Print and shaded views of the part. All mm, measured from the part's lowest x, y and z. Coordinates: 2 decimals unless noted, no trailing zeros. Loops run counter-clockwise (first coordinate to the right, second up) from the corner with the lowest first, then second, coordinate; pieces in that order, holes last. Notation, with made-up numbers: (39, -8.75) -> (58, -8.75) arc R14 cw to (58, -4.75) -> close; hole circle Ø10 at (-16.75, 38). An arc over 180 degrees is marked (long way). One line per item, written item: value. Start each with the question number.
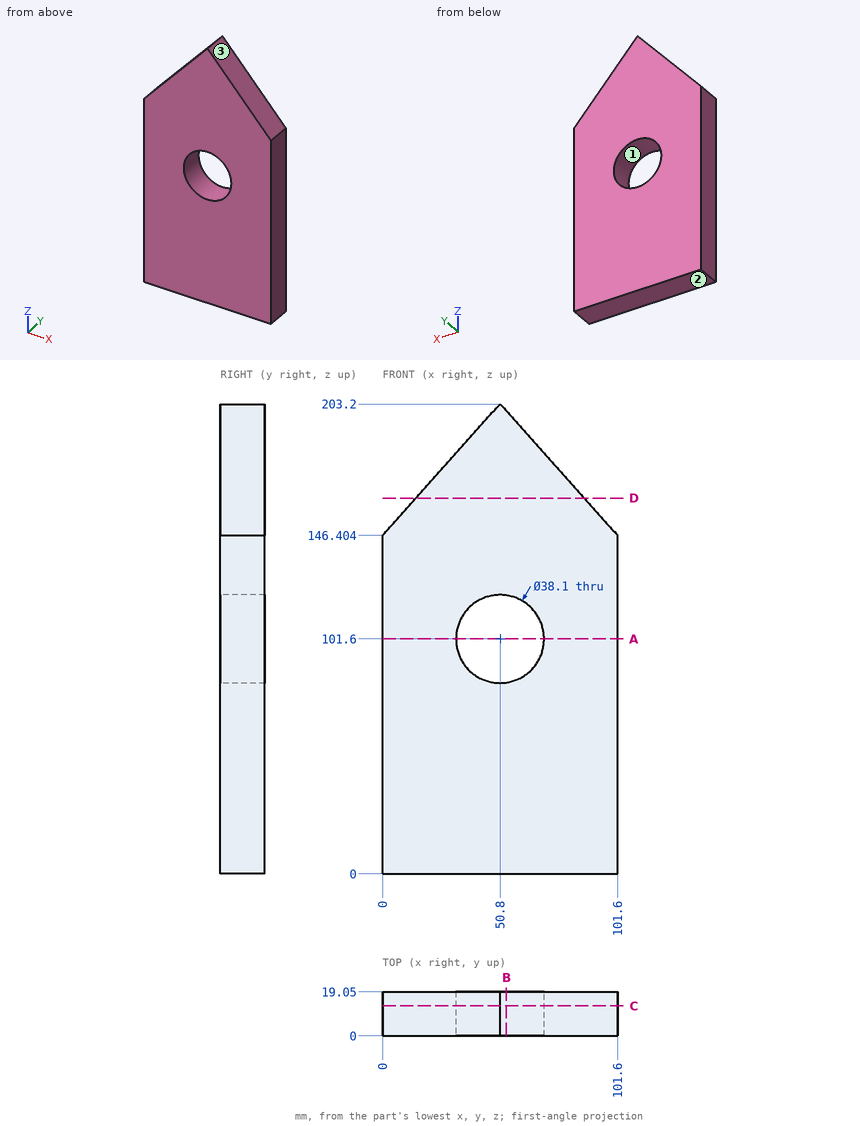
1) Pin check, flat tips, straight feed: pin 1 Ø10 at (x, y) = (60, 11.5) entering from +Z; pin 2 Ø12 at (x, z) = (25.5, 71.5) entering from -Y; pin 3 Ø1 at (x, y) = (49.5, 8) entering from +Z (1 decimal); pin 4 Ø8 at (y, z) = (3.5, 170) entering from -X. Stop position of each tip, or through.
2) Slice it at B-B (x = 53.5). Give the cut face in (y, z).
3) Slice it at C-C (y = 13). Give the cut face in (x, z).
4) Slice it at D-D (z = 162.5). Give the cut face in (x, y).
5) Probe line 1 (X direction, y = 3.5, z = 84.5) (1 decimal); line 2 (Z direction, x = 35, y = 11.5) (1 decimal); line 3 (Z direction, x = 36, y = 8.25) (1 decimal). List the from-to ranges inside material, lowest first. Write a range as from..to.
6) Pull direction Z, two halves, no side cores. Call the marked faces 1, 2 and 3: +Z half, -Z half, draft (parallel to the pull), parting line (faces both ways), or undercut.
7) Slice it at A-A (z = 101.6). Give the cut face in (x, y), then the cut area to 3 significant figures.
Check sheet entries:
1. pin 1: stops at z = 198.5
1. pin 2: stops at y = 0
1. pin 3: stops at z = 202.3
1. pin 4: stops at x = 17.53
2. outline: (0, 0) -> (19.05, 0) -> (19.05, 82.74) -> (0, 82.74) -> close; (0, 120.46) -> (19.05, 120.46) -> (19.05, 200.18) -> (0, 200.18) -> close
3. outline: (0, 0) -> (101.6, 0) -> (101.6, 146.4) -> (50.8, 203.2) -> (0, 146.4) -> close; hole circle Ø38.1 at (50.8, 101.6)
4. outline: (14.4, 0) -> (87.2, 0) -> (87.2, 19.05) -> (14.4, 19.05) -> close
5. line 1: x = 0..42.4, 59.2..101.6
5. line 2: z = 0..91, 112.2..185.5
5. line 3: z = 0..89.6, 113.6..186.7
6. face 1: undercut
6. face 2: -Z half
6. face 3: +Z half
7. outline: (0, 0) -> (31.75, 0) -> (31.75, 19.05) -> (0, 19.05) -> close; (69.85, 0) -> (101.6, 0) -> (101.6, 19.05) -> (69.85, 19.05) -> close
7. area: 1,210 mm^2
